The model under review builds one solid part; all positions refer to its coordinate system, in mm. Give positions to 0.01 mm unless a question says otherwise; leave off trailing zeros. Loops run counter-clockwise (first coordinate to the right, second up) from the corner with the lowest first, then second, coordinate; pieces in that order, holes last. Notation, with made-up numbers: M 11.5,61 L 59.5,61 A32 ccw 59.5,96 Z; hole C 41,1 d4. An arc over 180 degrees is marked long. Write item = value, one per line. Start each with the question number.
1. Wall thickness on line 1 along Y through (x, z) = (233, 797); line 2 along Z through (x, y) = (230, 3165); line 3 along Z through (x, y) = (249.5, 3131): over which ranges is each line inside the solid? List them lowest first. Write a range as from..to.
2. For pin 1 (2 mm diameter, centred on x = 316.5, y = 3152, fed in from -Z); pin 2 (5 mm diameter, centred on x = 240.5, z = 874.5, fed in from +Y); pin 3 (12 mm diameter, centred on x = 265, y = 3136.5, fed in from -Z); pin 4 (10 mm diameter, centred on y = 3155, z = 879, fed in from +X), all flat-tipped, find the tip position at first contact; note any pin that passes through.
3. We need section A-A on y = 3187. Give the boundary of the cut face in (x, z), then the cut area to 3 significant figures.
4. We need section B-B on x = 169. Give the boundary of the cut face in (y, z).
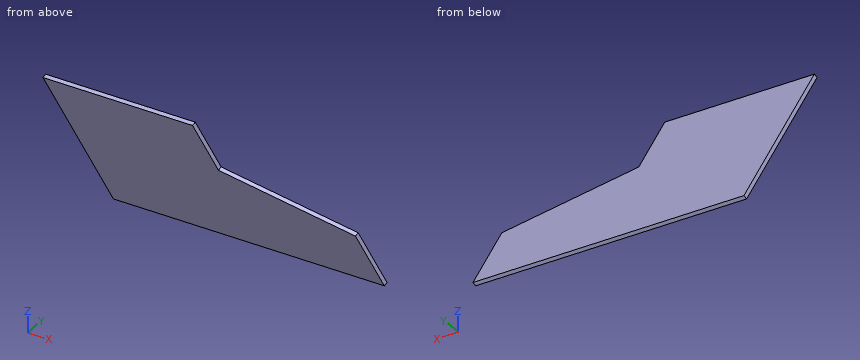
from build123d import *

# Parameters (mm, degrees)
BOSS_EXTRUDE1_DEPTH = 3


with BuildPart() as part:
    # Sketch1 → Boss-Extrude1 (new body)
    with BuildSketch(Plane(origin=(270.562015017, 2929.868417667, 1339.312972046), x_dir=(0.933919841, -0.218343191, 0.283054733), z_dir=(-0.093635076, -0.913565758, -0.395765181))):
        Polygon((-317.0861634, -434.442381086), (-183.365674706, -452.985058966), (-189.410130107, -496.574638387), (-84.476991235, -537.792492394), (-91.181057549, -586.138854741), (-199.742283926, -571.084947366), (-333.462772622, -552.542269486), align=None)
    extrude(amount=-BOSS_EXTRUDE1_DEPTH)


solid = part.part
Final values:
q1.line_1 = 3168.65..3171.94
q1.line_2 = 806.14..813.72
q1.line_3 = 880.01..887.59
q2.pin_1 = 813.37
q2.pin_2 = 3138.71
q2.pin_3 = 849.73
q2.pin_4 = through
q3.outline = M 145.43,782.95 L 146.73,775.06 L 180,767.19 L 196.04,770.97 Z
q3.area = 318 mm²
q4.outline = M 3140.39,877.38 L 3188.91,765.37 L 3191.7,766.51 L 3143.18,878.52 Z
